Could you check a few things on this model? Use its own coordinates, in mm. A direction names the side the tool comes from. Round coordinates to 2 decimals unless told otherwise and drop trailing zeros. Write each loop counter-clockwise with the first axis right and the second up, starting at its lowest first coordinate (ties: lowest second). Pieces come first, ordered by that corner, then holes. Notation, with made-up numbers: (-11.5, 83.5) - (31.5, 83.5) arc R22 ccw to (31.5, 94.5) - close; hole circle Ø1 at (-12.5, 40). An arc over 180 degrees is marked (long way). Put each result on its own line as item: value.
from build123d import *

# Parameters (mm, degrees)
SKETCH2_R           = 13.45
BOSS_EXTRUDE1_DEPTH = 48
SKETCH4_R           = 12
CUT_EXTRUDE1_DEPTH  = 48


with BuildPart() as part:
    # Sketch2 → Boss-Extrude1 (new body)
    with BuildSketch(Plane(origin=(0, 0, 0), x_dir=(1, 0, 0), z_dir=(0, 1, 0))):
        Polygon((-17.4, -17.4), (17.4, -17.4), (17.4, 0), (58.6, 25.6), (82.6, 25.6), (82.6, 29.6), (58.6, 29.6), (-17.4, 17.4), align=None)
        with Locations(Location((0, 0, 0), (0, 0, 270))):
            Circle(SKETCH2_R, mode=Mode.SUBTRACT)
    boss_extrude1 = extrude(amount=BOSS_EXTRUDE1_DEPTH)

    # Mirror1: Boss-Extrude1 across plane
    add(boss_extrude1.mirror(Plane(origin=(82.6, 0, 0), x_dir=(0, 0, 1), z_dir=(1, 0, 0))))

    # Sketch4 → Cut-Extrude1 (cut)
    with BuildSketch(Plane(origin=(0, 0, -29.6), x_dir=(-1, 0, 0), z_dir=(0, 0, -1))):
        with Locations((-82.6, 24)):
            Circle(SKETCH4_R)
        with BuildLine():
            Line((-101.6, 10.3), (-63.6, 10.3))
            ThreePointArc((-63.6, 10.3), (-61.85, 8.55), (-63.6, 6.8))
            Line((-63.6, 6.8), (-101.6, 6.8))
            ThreePointArc((-101.6, 6.8), (-103.35, 8.55), (-101.6, 10.3))
        make_face()
        with BuildLine():
            Line((-101.6, 37.7), (-63.6, 37.7))
            ThreePointArc((-63.6, 37.7), (-61.85, 39.45), (-63.6, 41.2))
            Line((-63.6, 41.2), (-101.6, 41.2))
            ThreePointArc((-101.6, 41.2), (-103.35, 39.45), (-101.6, 37.7))
        make_face()
    extrude(amount=-CUT_EXTRUDE1_DEPTH, mode=Mode.SUBTRACT)


solid = part.part
(1) Imagine slicing it at A-A, the plane y = 24. List the corners of the cut face in (x, z) for me.
Values found:
outline: (-17.4, -17.4) - (58.6, -29.6) - (70.6, -29.6) - (70.6, -25.6) - (58.6, -25.6) - (17.4, 0) - (17.4, 17.4) - (-17.4, 17.4) - close; (94.6, -29.6) - (106.6, -29.6) - (182.6, -17.4) - (182.6, 17.4) - (147.8, 17.4) - (147.8, 0) - (106.6, -25.6) - (94.6, -25.6) - close; hole circle Ø26.9 at (0, 0); hole circle Ø26.9 at (165.2, 0)
(2) I'm going to push flat-ended pins straight in: pin 1 (2 mm diameter, centred on x = 128.5, y = 17.5, fed in from -Z) (3 decimals); pin 2 (6 mm diameter, centred on x = 55.5, y = 34.5, fed in from +Z); pin 3 (12 mm diameter, centred on x = 17.5, y = 19.5, fed in from +Z); pin 4 (5 mm diameter, centred on x = 36.5, y = 36.5, fed in from -Z). Where does each tip first touch, or does it pass through?
Values found:
pin 1: stops at z = -26.245
pin 2: stops at z = -21.81
pin 3: stops at z = 17.4
pin 4: stops at z = -26.45
(3) Imagine slicing it at C-C, the plane z = -20. List the corners of the cut face in (x, y) for me.
Values found:
outline: (-1.2, 0) - (49.59, 0) - (49.59, 48) - (-1.2, 48) - close; (115.61, 0) - (166.4, 0) - (166.4, 48) - (115.61, 48) - close
(4) For faces 1 (the face through (82, 41.2, -28)), 2 (the face through (151.864, 23.664, -1.751)), 3 (the face through (147.8, 24, 9)), which set-ups out of +Z, -Z, +X, -X, +Y, -Y let a thin tool reach every point of the face, with its end or its side?
Values found:
face 1: +Z, -Z
face 2: +Y, -Y
face 3: +Z, +Y, -Y
(5) If we mould it in two halves opening along X, with no side actions, what happens to faces 4 (the face through (0, 24, 17.4)), 5 (the face through (61.85, 39.41, -27.63)), 6 (the face through (144.068, 23.664, -23.585))? For each: pulls with the +X half, pulls with the -X half, needs draft (parallel to the pull), parting line crosses it, or undercut.
Values found:
face 4: needs draft
face 5: undercut
face 6: pulls with the +X half
(6) Imagine slicing it at D-D, the plane y = 44. List the corners of the cut face in (x, z) for me.
Values found:
outline: (-17.4, -17.4) - (58.6, -29.6) - (106.6, -29.6) - (182.6, -17.4) - (182.6, 17.4) - (147.8, 17.4) - (147.8, 0) - (106.6, -25.6) - (58.6, -25.6) - (17.4, 0) - (17.4, 17.4) - (-17.4, 17.4) - close; hole circle Ø26.9 at (0, 0); hole circle Ø26.9 at (165.2, 0)
(7) Please list where these lines run through material, in increasing order: probe 1 along X at (y, z) = (29, 0); probe 2 along Y at (x, z) = (82.6, -27.5); probe 3 along X at (y, z) = (36, 6.5). Write a range as from..to.
Values found:
probe 1: x = -17.4..-13.45, 13.45..17.4, 147.8..151.75, 178.65..182.6
probe 2: y = 0..6.8, 10.3..12, 36..37.7, 41.2..48
probe 3: x = -17.4..-11.78, 11.78..17.4, 147.8..153.42, 176.98..182.6
(8) Imagine slicing it at B-B, the plane x = 82.6. List the corners of the cut face in (y, z) for me, then the cut area to 3 significant figures.
Values found:
outline: (0, -29.6) - (6.8, -29.6) - (6.8, -25.6) - (0, -25.6) - close; (10.3, -29.6) - (12, -29.6) - (12, -25.6) - (10.3, -25.6) - close; (36, -29.6) - (37.7, -29.6) - (37.7, -25.6) - (36, -25.6) - close; (41.2, -29.6) - (48, -29.6) - (48, -25.6) - (41.2, -25.6) - close
area: 68.0 mm^2
